from build123d import *

# Parameters (mm, degrees)
BOSS_EXTRUDE1_DEPTH = 25
SKETCH2_R           = 3.175
CUT_EXTRUDE1_DEPTH  = 40


with BuildPart() as part:
    # Sketch1 → Boss-Extrude1 (new body)
    with BuildSketch(Plane.XY):
        Polygon((0, 0), (19.584, 0), (19.584, 104.78), (0, 104.78), (0, 80.95), (6.27, 80.95), (6.27, 24.23), (0, 24.23), align=None)
    extrude(amount=BOSS_EXTRUDE1_DEPTH)

    # Sketch2 → Cut-Extrude1 (cut)
    with BuildSketch(Plane(origin=(0, 0, 0), x_dir=(0, 0, -1), z_dir=(1, 0, 0))):
        with Locations(Location((-12.5, 92.28, 0), (0, 0, 270))):
            Circle(SKETCH2_R)
        with Locations(Location((-12.5, 12.5, 0), (0, 0, 270))):
            Circle(SKETCH2_R)
    extrude(amount=CUT_EXTRUDE1_DEPTH, mode=Mode.SUBTRACT)


solid = part.part
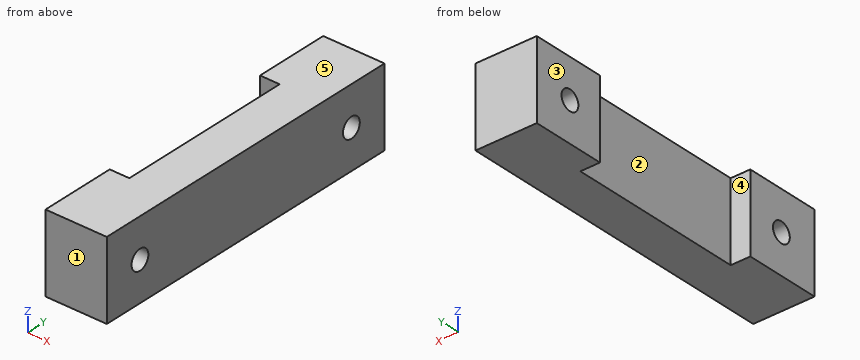
Build history of the part. All positions in model axes, mm. Face numbers are marked on the shaded views. A direction names the side the tool comes from. Give positions to 0.01 mm unless a question says otherwise; leave off trailing zeros. Order: outer loops, then holes, each group sorted by start corner. A loop starts at its lowest first (then second) coordinate and runs counter-clockwise, first axis right, second up. Notation, with made-up numbers: M 85,78 L 121,78 A12 cw 121,91 Z; hole C 27,67 d6. An arc over 180 degrees is marked long. Use one line per item in the form item = value.
1) Saw through at A-A (z = 12.5). Give the cut face in (x, y) (3 decimals).
Calculated:
outline = M 0,0 L 19.584,0 L 19.584,9.325 L 0,9.325 Z; M 0,15.675 L 19.584,15.675 L 19.584,89.105 L 0,89.105 L 0,80.95 L 6.27,80.95 L 6.27,24.23 L 0,24.23 Z; M 0,95.455 L 19.584,95.455 L 19.584,104.78 L 0,104.78 Z
2) Two-plate mould, pull along Y, no slides. Class the marked faces 1, 2 and 3: released by +Y, released by -Y, zero draft, split by the parting line, or undercut.
Calculated:
face_1 = released by -Y
face_2 = undercut
face_3 = zero draft
3) Saw through at D-D (x = 11.25). Give the cut face in (y, z) (3 decimals).
Calculated:
outline = M 0,0 L 104.78,0 L 104.78,25 L 0,25 Z; hole C 12.5,12.5 d6.35; hole C 92.28,12.5 d6.35
4) Saw through at C-C (y = 92.28). Give the cut face in (x, z) (3 decimals), plus the area to 3 significant figures.
Calculated:
outline = M 0,0 L 19.584,0 L 19.584,9.325 L 0,9.325 Z; M 0,15.675 L 19.584,15.675 L 19.584,25 L 0,25 Z
area = 365 mm2
5) Saw through at B-B (x = 4.5). Give the cut face in (y, z) (3 decimals), plus the area to 3 significant figures.
Calculated:
outline = M 0,0 L 24.23,0 L 24.23,25 L 0,25 Z; M 80.95,0 L 104.78,0 L 104.78,25 L 80.95,25 Z; hole C 12.5,12.5 d6.35; hole C 92.28,12.5 d6.35
area = 1,140 mm2
6) Probe probe 1 along Y at (x, z) = (13, 12.5) (3 decimals); probe 2 along Y at (x, z) = (5, 12.5) (3 decimals); probe 3 along Y at (x, z) = (1, 5.5). List the from-to ranges inside material, lowest first.
Calculated:
probe_1 = 0 to 9.325, 15.675 to 89.105, 95.455 to 104.78
probe_2 = 0 to 9.325, 15.675 to 24.23, 80.95 to 89.105, 95.455 to 104.78
probe_3 = 0 to 24.23, 80.95 to 104.78
7) Drop a flat-ended pin along its axis: pin 1 (2 mm diameter, centred on y = 44, z = 20, fed in from -X). Give the stop position or say it passes through.
Calculated:
pin_1 = 6.27
8) Tool access for the marked faces 4 and 5: list every direction of +Z, -Z, +X, -X, +Y, -Y with a clear straight run to the whole face (end or side of a thin tool).
Calculated:
face_4 = +Z, -Z, -X
face_5 = +Z, +X, -X, +Y, -Y
